The listing builds one solid part. Answer for the finished solid, in the listing's coordinates (mm). Give positions to 0.01 mm unless a question says otherwise; leave off trailing zeros. Order: outer loops, then holes, each group sorted by start corner. A loop starts at its lowest first (then second) coordinate and runs counter-clockwise, first axis right, second up. Notation, with made-up numbers: (-21, 43) - (14, 43) arc R6 ccw to (14, 53) - close; hole circle Ø3 at (73.25, 61). An arc over 180 degrees is marked (long way). Answer in a Markdown table with one row per item.
Autodesk Inventor part; units mm, degrees
ref_plane "YZ Plane" through (0, 0, 0) normal (1, 0, 0) x (0, 1, 0)
ref_plane "XZ Plane" through (0, 0, 0) normal (0, 1, 0) x (-1, 0, 0)
ref_plane "XY Plane" through (0, 0, 0) normal (0, 0, 1) x (1, 0, 0)
sketch "Sketch1" plane through (0, 0, 0) normal (0, 0, 1) x (1, 0, 0)
  line L0 (0, 110.6854) -> (-127, 110.6854)
  line L1 (-127, 110.6854) -> (-127, -143.3146)
  line L2 (-127, -143.3146) -> (0, -143.3146)
  line L3 (-127, 110.6854) -> (127, 110.6854)
  line L4 (-127, -143.3146) -> (-127, 110.6854)
  line L5 (127, -143.3146) -> (-127, -143.3146)
  line L6 (127, 110.6854) -> (127, -143.3146)
  line L7 (0, 110.6854) -> (127, 110.6854)
  line L8 (127, 110.6854) -> (127, -143.3146)
  line L9 (127, -143.3146) -> (0, -143.3146)
  circle A0 centre (15.4948, -84.6086) radius 1.3281
  circle A1 centre (0, -100.1034) radius 10.5
  circle A2 centre (-15.4948, -115.5982) radius 1.3281
  circle A3 centre (-15.4948, -84.6086) radius 1.3281
  circle A4 centre (15.4948, -115.5982) radius 1.3281
  circle A5 centre (-113.85, -97.5687) radius 2.5
  circle A6 centre (-77.85, -97.5687) radius 2.5
  circle A7 centre (-95.85, -79.5687) radius 2.5
  circle A8 centre (-95.85, -115.5687) radius 2.5
  point P0 (0, 0)
  point P1 (29.6393, -143.3146)
  point P2 (-29.6393, -143.3146)
  dimension "d0" = 254
  dimension "d1" = 127
extrude "Extrusion1" add sketch "Sketch1" along normal blind 3.175 contours L3 L6 L5 L2 L1 L0 | A0 | A1 | A2 | A3 | A4 | A5 | A6 | A7 | A8
sketch "Sketch3" plane through (0, 0, 0) normal (0, 0, -1) x (-1, 0, 0)
  circle A0 centre (0, -100.1034) radius 10.5
  spline S0 degree 2 number of poles 163
  spline S1 degree 2 number of poles 163
  spline S2 degree 2 number of poles 163
  spline S3 degree 2 number of poles 163
  circle A1 centre (-15.4948, -84.6086) radius 1.3281
  circle A2 centre (15.4948, -84.6086) radius 1.3281
  circle A3 centre (15.4948, -115.5982) radius 1.3281
  circle A4 centre (-15.4948, -115.5982) radius 1.3281
  point P0 (0, 0)
  point P1 (-15.4948, -83.0805)
  point P2 (-16.4994, -85.7601)
extrude "Extrusion3" cut sketch "Sketch3" against normal up to surface (3.175 mm away)
sketch "Sketch4" plane through (0, 0, 0) normal (0, 0, -1) x (-1, 0, 0)
  circle A0 centre (110.85, -124.0687) radius 2.5
  circle A1 centre (78.1, -71.0687) radius 2.5
  circle A2 centre (113.5793, -71.0687) radius 2.5
  circle A3 centre (110.85, -124.0687) radius 2.5
  circle A4 centre (95.85, -124.0687) radius 2.5
  circle A5 centre (80.85, -124.0687) radius 2.5
  line L0 (117.35, -68.0687) -> (117.35, -127.0687)
  line L1 (111.8085, -66.0687) -> (115.35, -66.0687)
  line L2 (109.8085, -68.0687) -> (109.8085, -76.5687)
  line L3 (109.8085, -76.5687) -> (112.4358, -76.5687)
  arc A6 (113.1429, -76.8616) -> (112.4358, -76.5687) centre (112.4358, -77.5687) ccw
  line L4 (113.1429, -76.8616) -> (116.5571, -80.2758)
  arc A7 (116.85, -80.9829) -> (116.5571, -80.2758) centre (115.85, -80.9829) ccw
  line L5 (116.85, -80.9829) -> (116.85, -83.3972)
  line L6 (116.85, -83.3972) -> (116.4142, -82.9614)
  arc A8 (117, -84.3756) -> (116.4142, -82.9614) centre (115, -84.3756) ccw
  line L7 (117, -84.3756) -> (117, -110.7619)
  arc A9 (116.4142, -112.1761) -> (117, -110.7619) centre (115, -110.7619) ccw
  line L8 (116.4142, -112.1761) -> (116.85, -111.7403)
  line L9 (116.85, -111.7403) -> (116.85, -114.1545)
  arc A10 (116.5571, -114.8616) -> (116.85, -114.1545) centre (115.85, -114.1545) ccw
  line L10 (116.5571, -114.8616) -> (113.1429, -118.2758)
  arc A11 (112.4358, -118.5687) -> (113.1429, -118.2758) centre (112.4358, -117.5687) ccw
  line L11 (112.4358, -118.5687) -> (110.0216, -118.5687)
  line L12 (110.0216, -118.5687) -> (110.4574, -118.1329)
  arc A12 (109.0431, -118.7187) -> (110.4574, -118.1329) centre (109.0431, -116.7187) ccw
  line L13 (109.0431, -118.7187) -> (82.6569, -118.7187)
  arc A13 (81.8969, -118.5687) -> (82.6569, -118.7187) centre (82.6569, -116.7187) ccw
  line L14 (81.8969, -118.5687) -> (79.2642, -118.5687)
  arc A14 (78.5571, -118.2758) -> (79.2642, -118.5687) centre (79.2642, -117.5687) ccw
  line L15 (78.5571, -118.2758) -> (75.1429, -114.8616)
  arc A15 (74.85, -114.1545) -> (75.1429, -114.8616) centre (75.85, -114.1545) ccw
  line L16 (74.85, -114.1545) -> (74.85, -111.5218)
  arc A16 (74.7, -110.7619) -> (74.85, -111.5218) centre (76.7, -110.7619) ccw
  line L17 (74.7, -110.7619) -> (74.7, -84.3756)
  arc A17 (74.85, -83.6157) -> (74.7, -84.3756) centre (76.7, -84.3756) ccw
  line L18 (74.85, -83.6157) -> (74.85, -80.9829)
  arc A18 (75.1429, -80.2758) -> (74.85, -80.9829) centre (75.85, -80.9829) ccw
  line L19 (75.1429, -80.2758) -> (78.5571, -76.8616)
  arc A19 (79.2642, -76.5687) -> (78.5571, -76.8616) centre (79.2642, -77.5687) ccw
  line L20 (79.2642, -76.5687) -> (81.8915, -76.5687)
  line L21 (81.8915, -76.5687) -> (81.8915, -76.0687)
  line L22 (81.8915, -76.0687) -> (81.85, -76.0687)
  line L23 (81.85, -68.0687) -> (81.85, -76.0687)
  line L24 (76.35, -66.0687) -> (79.85, -66.0687)
  line L25 (74.35, -127.0687) -> (74.35, -68.0687)
  line L26 (115.35, -129.0687) -> (76.35, -129.0687)
  circle A20 centre (80.85, -124.0687) radius 2.5
  circle A21 centre (113.5793, -71.0687) radius 2.5
  circle A22 centre (78.1, -71.0687) radius 2.5
  arc A23 (115.35, -129.0687) -> (117.35, -127.0687) centre (115.35, -127.0687) ccw
  arc A24 (117.35, -68.0687) -> (115.35, -66.0687) centre (115.35, -68.0687) ccw
  arc A25 (111.8085, -66.0687) -> (109.8085, -68.0687) centre (111.8085, -68.0687) ccw
  arc A26 (81.85, -68.0687) -> (79.85, -66.0687) centre (79.85, -68.0687) ccw
  arc A27 (76.35, -66.0687) -> (74.35, -68.0687) centre (76.35, -68.0687) ccw
  arc A28 (74.35, -127.0687) -> (76.35, -129.0687) centre (76.35, -127.0687) ccw
  point P0 (0, 0)
extrude "Extrusion4" cut sketch "Sketch4" against normal up to surface (3.175 mm away) contours A0 | A1 | A2 | A4 | A5
sketch "Sketch5" plane through (0, 0, 3.175) normal (0, 0, 1) x (1, 0, 0)
  circle A0 centre (-113.85, -97.5687) radius 2.5
  circle A1 centre (-77.85, -97.5687) radius 2.5
  circle A2 centre (-95.85, -79.5687) radius 2.5
  circle A3 centre (-95.85, -115.5687) radius 2.5
  circle A4 centre (15.4948, -84.6086) radius 1.3281
  circle A5 centre (0, -100.1034) radius 10.5
  circle A6 centre (-15.4948, -115.5982) radius 1.3281
  circle A7 centre (-15.4948, -84.6086) radius 1.3281
  circle A8 centre (15.4948, -115.5982) radius 1.3281
  line L0 (-127, 110.6854) -> (127, 110.6854)
  line L1 (-127, -143.3146) -> (-127, 110.6854)
  line L2 (127, -143.3146) -> (-127, -143.3146)
  line L3 (127, 110.6854) -> (127, -143.3146)
  circle A9 centre (-113.85, -97.5687) radius 2.5
  circle A10 centre (-77.85, -97.5687) radius 2.5
  circle A11 centre (-95.85, -79.5687) radius 2.5
  circle A12 centre (-95.85, -115.5687) radius 2.5
  circle A13 centre (15.4948, -84.6086) radius 1.3281
  circle A14 centre (0, -100.1034) radius 10.5
  circle A15 centre (-15.4948, -115.5982) radius 1.3281
  circle A16 centre (-15.4948, -84.6086) radius 1.3281
  circle A17 centre (15.4948, -115.5982) radius 1.3281
  line L4 (-127, 110.6854) -> (127, 110.6854)
  line L5 (-127, -143.3146) -> (-127, 110.6854)
  line L6 (127, -143.3146) -> (-127, -143.3146)
  line L7 (127, 110.6854) -> (127, -143.3146)
  circle A18 centre (-113.85, -97.5687) radius 2.5
  circle A19 centre (-77.85, -97.5687) radius 2.5
  circle A20 centre (-95.85, -79.5687) radius 2.5
  circle A21 centre (-95.85, -115.5687) radius 2.5
  circle A22 centre (15.4948, -84.6086) radius 1.3281
  circle A23 centre (0, -100.1034) radius 10.5
  circle A24 centre (-15.4948, -115.5982) radius 1.3281
  circle A25 centre (-15.4948, -84.6086) radius 1.3281
  circle A26 centre (15.4948, -115.5982) radius 1.3281
  line L8 (-127, 110.6854) -> (127, 110.6854)
  line L9 (-127, -143.3146) -> (-127, 110.6854)
  line L10 (127, -143.3146) -> (-127, -143.3146)
  line L11 (127, 110.6854) -> (127, -143.3146)
  circle A27 centre (-113.85, -97.5687) radius 2.5
  circle A28 centre (-77.85, -97.5687) radius 2.5
  circle A29 centre (-95.85, -79.5687) radius 2.5
  circle A30 centre (-95.85, -115.5687) radius 2.5
  circle A31 centre (15.4948, -84.6086) radius 1.3281
  circle A32 centre (0, -100.1034) radius 10.5
  circle A33 centre (-15.4948, -115.5982) radius 1.3281
  circle A34 centre (-15.4948, -84.6086) radius 1.3281
  circle A35 centre (15.4948, -115.5982) radius 1.3281
  line L12 (-127, 110.6854) -> (127, 110.6854)
  line L13 (-127, -143.3146) -> (-127, 110.6854)
  line L14 (127, -143.3146) -> (-127, -143.3146)
  line L15 (127, 110.6854) -> (127, -143.3146)
  circle A36 centre (-113.85, -97.5687) radius 2.5
  circle A37 centre (-77.85, -97.5687) radius 2.5
  circle A38 centre (-95.85, -79.5687) radius 2.5
  circle A39 centre (-95.85, -115.5687) radius 2.5
  circle A40 centre (15.4948, -84.6086) radius 1.3281
  circle A41 centre (0, -100.1034) radius 10.5
  circle A42 centre (-15.4948, -115.5982) radius 1.3281
  circle A43 centre (-15.4948, -84.6086) radius 1.3281
  circle A44 centre (15.4948, -115.5982) radius 1.3281
  line L16 (-127, 110.6854) -> (127, 110.6854)
  line L17 (-127, -143.3146) -> (-127, 110.6854)
  line L18 (127, -143.3146) -> (-127, -143.3146)
  line L19 (127, 110.6854) -> (127, -143.3146)
  line L20 (-95.85, -97.5687) -> (-44.7057, -11.637)
  line L21 (-95.85, -97.5687) -> (4.15, -97.5687) construction
  point P0 (0, 0)
  dimension "d11" = 100
  dimension "d12" = 59.24
properties part number "LeftAlPanel" material "Aluminum 6061"
Item 1: Consider line 1 (X direction, y = -123.5, z = 2.45); line 2 (X direction, y = -83.5, z = 0.6); line 3 (X direction, y = -69, z = 1.25). Determine where each line is inside the solid, lowest interval first.
Answer block:
| item | result |
|---|---|
| line 1 | -127 to -113.28, -108.42 to -98.28, -93.42 to -83.28, -78.42 to 127 |
| line 2 | -127 to -16.23, -14.76 to 14.76, 16.23 to 127 |
| line 3 | -127 to -114.98, -112.18 to -79.5, -76.7 to 127 |
Item 2: Each of these flat-tipped pins is pushed along its axis until it touches: P1, Ø3, axis at x = -78.1, y = -71.07, coming from the +Z side; P2, Ø6.5, axis at x = -110.85, y = -124.07, coming from the +Z side (3 decimals). Where does it stop, or does it pass through?
Answer block:
| item | result |
|---|---|
| P1 | through |
| P2 | z = 3.175 |
Item 3: Determine the mould class of faces 1 (the face through (-2, -15, 3.175)), 2 (the face through (1.367, -89.693, 1.565)) for opening direction X: pulls with the +X half, pulls with the -X half, needs draft (parallel to the pull), parting line crosses it, or undercut.
Answer block:
| item | result |
|---|---|
| face 1 | needs draft |
| face 2 | undercut |
Item 4: Find section A-A on x = 0. Write down the section's boundary in (y, z) (3 decimals).
Answer block:
| item | result |
|---|---|
| outline | (-143.315, 0) - (-110.603, 0) - (-110.603, 3.175) - (-143.315, 3.175) - close; (-89.603, 0) - (110.685, 0) - (110.685, 3.175) - (-89.603, 3.175) - close |
